```python
from build123d import *

# Parameters (mm, degrees)
F0_W      = 62.3333714902
F0_H      = 74.1953216493
F1_DEPTH  = 7.62
F3_DEPTH  = 25.4
F4_DEPTH  = 33.02
F5_W      = 62.3333714902
F5_H      = 7.3264986277
F6_DEPTH  = 45.72
F8_DEPTH  = 25.4
F9_W      = 6.5124388784
F9_H      = 29.771162197
F10_DEPTH = 45.72
F12_DEPTH = 25.4
F13_W     = 9.0668685734
F13_H     = 37.0976608247
F14_DEPTH = 45.72


with BuildPart() as f1:
    # F0 (on Top) → F1 (new body)
    with BuildSketch(Plane.XY):
        with Locations((-0.1162942499, -1.7444025725)):
            Rectangle(F0_W, F0_H)
    extrude(amount=F1_DEPTH)

    # F2 (on face) → F3 (join)
    with BuildSketch(Plane.XY.offset(7.62)):
        Polygon((-31.282979995, 35.3532582521), (-31.282979995, -1.7444025725), (0, 35.3532582521), align=None)
    extrude(amount=F3_DEPTH)

    # F4 (cut): a face of the model
    f4_faces = [f1.faces().sort_by_distance(p)[0] for p in [
        (-20.8553199967, 22.9873713106, 33.02),
    ]]
    extrude(f4_faces, amount=-F4_DEPTH, mode=Mode.SUBTRACT)

    # F5 (on face) → F6 (join)
    with BuildSketch(Plane.XY.offset(7.62)):
        with Locations((-0.1162942499, -5.4076518863)):
            Rectangle(F5_W, F5_H)
    extrude(amount=F6_DEPTH)

    # F7 (on face) → F8 (cut)
    with BuildSketch(Plane.XZ.offset(9.0709012002)):
        Polygon((-31.282979995, 53.34), (-31.282979995, 7.62), (31.0503914952, 53.34), align=None)
    extrude(amount=-F8_DEPTH, mode=Mode.SUBTRACT)

    # F9 (on face) → F10 (join)
    with BuildSketch(Plane.XY.offset(7.62)):
        with Locations((27.794172056, -23.9564822987)):
            Rectangle(F9_W, F9_H)
    extrude(amount=F10_DEPTH)

    # F11 (on face) → F12 (cut)
    with BuildSketch(Plane(origin=(24.5379526168, 0, 0), x_dir=(0, -1, 0), z_dir=(-1, 0, 0))):
        Polygon((38.8420633972, 53.34), (9.0709012002, 53.34), (38.8420633972, 7.62), align=None)
    extrude(amount=-F12_DEPTH, mode=Mode.SUBTRACT)

    # F13 (on face) → F14 (join)
    with BuildSketch(Plane.XY.offset(7.62)):
        with Locations((26.5169572085, 16.8044278398)):
            Rectangle(F13_W, F13_H)
    extrude(amount=F14_DEPTH)


solid = f1.part
```
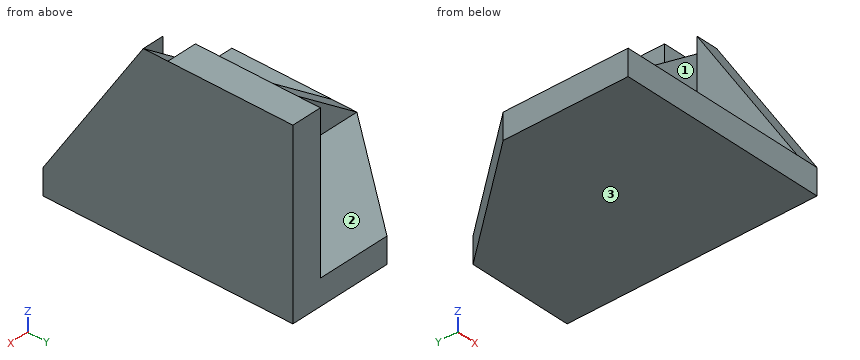
Could you check a few things on this model? Use its own coordinates, in mm. Face numbers are marked on the shaded views. A direction names the side the tool comes from. Round coordinates to 2 decimals unless told otherwise and drop trailing zeros. Loops run counter-clockwise (first coordinate to the right, second up) from the corner with the lowest first, then second, coordinate; pieces in that order, holes last. Notation, with made-up numbers: (31, -14.75) -> (55, -14.75) arc R33 cw to (55, 14.25) -> close; hole circle Ø2 at (10, 62). An arc over 180 degrees is marked (long way). One line per question, with ' | ' between items.
(1) For pin 1 Ø3 at (x, y) = (-20.5, -6) entering from +Z; pin 2 Ø4 at (x, z) = (-4, 28.5) entering from -Y; pin 3 Ø8 at (x, z) = (1, 29) entering from +Y, each with a flat end and sliding along its axis, tell me the tip position at first contact or that it passes through.
Model answer:
pin 1: stops at z = 16.63 | pin 2: stops at y = -9.07 | pin 3: stops at y = -1.74
(2) If we section it at D-D on y = -21: List the corners of the cut face in (x, z) for me, and give its area (3 significant figures).
Model answer:
outline: (-31.28, 0) -> (31.05, 0) -> (31.05, 35.02) -> (24.54, 35.02) -> (24.54, 7.62) -> (-31.28, 7.62) -> close | area: 653 mm^2
(3) For the marked faces 1, 2 and 3, which set-ups out of +Z, -Z, +X, -X, +Y, -Y let a thin tool reach every point of the face, with its end or its side?
Model answer:
face 1: +Z, -X, -Y | face 2: +Z, -X, +Y | face 3: -Z, +X, -X, +Y, -Y
(4) If we section it at A-A on x = 12: List the corners of the cut face in (y, z) for me.
Model answer:
outline: (-38.84, 0) -> (35.35, 0) -> (35.35, 7.62) -> (-1.74, 7.62) -> (-1.74, 39.37) -> (-9.07, 39.37) -> (-9.07, 7.62) -> (-38.84, 7.62) -> close
(5) If we section it at C-C on y = -31: List the corners of the cut face in (x, z) for me.
Model answer:
outline: (-31.28, 0) -> (31.05, 0) -> (31.05, 19.66) -> (24.54, 19.66) -> (24.54, 7.62) -> (-31.28, 7.62) -> close
(6) If I drill on probe 1 along Z at (x, y) = (-18, 6); probe 2 along Y at (x, z) = (15, 35); probe 3 along X at (y, z) = (6, 19), over which ranges is the centre line in solid material (lowest first)?
Model answer:
probe 1: z = 0 to 7.62 | probe 2: y = -9.07 to -1.74 | probe 3: x = 21.98 to 31.05
(7) If we section it at B-B on z = 41.5: List the corners of the cut face in (x, y) for me.
Model answer:
outline: (14.91, -9.07) -> (24.54, -9.07) -> (24.54, -16.78) -> (31.05, -16.78) -> (31.05, 35.35) -> (21.98, 35.35) -> (21.98, -1.74) -> (14.91, -1.74) -> close
